CAD build for the part. Positions are in the model's coordinates, mm. A direction names the side the tool comes from. Give positions to 0.01 mm unless a question says otherwise; leave off trailing zeros. Order: outer loops, then holes, each group sorted by start corner. A loop starts at its lowest first (then second) coordinate and runs counter-clockwise, first axis right, second up.
```python
from build123d import *

# Parameters (mm, degrees)
F0_W     = 52
F0_H     = 42
F0_W_2   = 46
F0_H_2   = 36
F0_W_3   = 22
F0_H_3   = 10
F1_DEPTH = 5
F2_DEPTH = 30


with BuildPart() as f1:
    # F0 (on Front) → F1 (new body)
    with BuildSketch(Plane.XZ):
        with Locations((23, 18)):
            Rectangle(F0_W, F0_H)
        with Locations((23, 18)):
            Rectangle(F0_W_2, F0_H_2, mode=Mode.SUBTRACT)
        with Locations((23, 18)):
            Rectangle(F0_W_2, F0_H_2)
        with Locations((26, 15)):
            Rectangle(F0_W_3, F0_H_3, mode=Mode.SUBTRACT)
    extrude(amount=-F1_DEPTH)

    # F0 (on Front) → F2 (join)
    with BuildSketch(Plane.XZ):
        with Locations((23, 18)):
            Rectangle(F0_W, F0_H)
        with Locations((23, 18)):
            Rectangle(F0_W_2, F0_H_2, mode=Mode.SUBTRACT)
    extrude(amount=F2_DEPTH)


solid = f1.part
```
Item 1: Drop a flat-ended pin along its axis: pin 1 Ø6 at (x, z) = (35.5, 29) entering from -Y. Give the stop position or say it passes through.
Item 2: Slice it at C-C (z = 16). Give the cut face in (x, y).
Item 3: Slice it at A-A (x = 26). Give the cut face in (y, z).
Item 4: Two-plate mould, pull along X, no slides. Class faces 1 (the face through (23, 5, 23)), 2 (the face through (-3, -12, 18)), 3 (the face through (49, -12, 18)), 4 (the face through (46, -15, 18)): released by +X, released by -X, zero draft, split by the parting line, or undercut.
Item 5: Slice it at D-D (z = 4.5). Give the cut face in (x, y), and give its area (3 significant figures).
Item 6: Wall check: L1, parallel to Z at x = 15, y = -18; L2, parallel to X at y = 0.5, z = 19; L3, parallel to Z at x = 31, y = 1. Give the ranges that are in metal, low to high.
Item 7: Tool access for faces 5 (the face through (23, -15, 0)), 6 (the face through (26, 2, 10)), 7 (the face through (17, -30, -1)): list every direction of +Z, -Z, +X, -X, +Y, -Y with a clear straight run to the whole face (end or side of a thin tool).
Item 8: Slice it at B-B (y = 2). Give the cut face in (x, z), and give its area (3 significant figures).
A:
1. pin 1: stops at y = 0
2. outline: (-3, -30) - (0, -30) - (0, 0) - (15, 0) - (15, 5) - (-3, 5) - close; (37, 0) - (46, 0) - (46, -30) - (49, -30) - (49, 5) - (37, 5) - close
3. outline: (-30, -3) - (5, -3) - (5, 10) - (0, 10) - (0, 0) - (-30, 0) - close; (-30, 36) - (0, 36) - (0, 20) - (5, 20) - (5, 39) - (-30, 39) - close
4. face 1: zero draft
4. face 2: released by -X
4. face 3: released by +X
4. face 4: undercut
5. outline: (-3, -30) - (0, -30) - (0, 0) - (46, 0) - (46, -30) - (49, -30) - (49, 5) - (-3, 5) - close
5. area: 440 mm2
6. L1: z = -3 to 0, 36 to 39
6. L2: x = -3 to 15, 37 to 49
6. L3: z = -3 to 10, 20 to 39
7. face 5: -Y
7. face 6: +Y, -Y
7. face 7: +Z, -Z, +X, -X, -Y
8. outline: (-3, -3) - (49, -3) - (49, 39) - (-3, 39) - close; hole (15, 10) - (37, 10) - (37, 20) - (15, 20) - close
8. area: 1,960 mm2
